The drawing under review shows one solid part. Ordinate dimensions are in mm from its lowest x, y, z. A direction names the side the tool comes from. Give positions to 0.01 mm unless a question says otherwise; leave off trailing zeros. Loops run counter-clockwise (first coordinate to the right, second up) from the corner with the lowest first, then second, coordinate; pieces in that order, holes last. Notation, with made-up numbers: (38.25, 62.25) -> (90.25, 62.25) arc R26 ccw to (90.25, 100.25) -> close; hole circle Ø6 at (-21.5, 8). An arc over 180 degrees is marked (long way). Answer in a Markdown table with one row per item. Add a question column.
(1) Consider section C-C on z = 15.75. Write out the cut boundary in (x, y), then the cut area to 4 significant figures.
(2) For the marked faces 1 and 2, list the 3-axis set-ups (+Z, -Z, +X, -X, +Y, -Y) from which the entire face can be reached by the end or side of a thin tool; tool diameter is ignored.
(3) Consider section D-D on y = 77.5. Write out the cut boundary in (x, z), then the cut area to 3 significant figures.
(4) For pin 1 (19 mm diameter, centred on x = 47, y = 59.5, fed in from +Z); pin 2 (2.5 mm diameter, centred on x = 18, z = 3.5, fed in from -Y); pin 3 (10.5 mm diameter, centred on y = 94, z = 6, fed in from +X), all flat-tipped, find the tip position at first contact; note any pin that passes through.
(5) For line 1 (X direction, y = 70.5, z = 14.5); line 2 (X direction, y = 79, z = 1.5); line 3 (Y direction, x = 19, z = 1.25), list the stretches that pass through material, from the lowest coordinate up.
(6) Draft analysis for pull direction X (two halves, no side actions). For the marked faces 3, 4 and 5, state which applies: +X half, -X half, draft (parallel to the pull), parting line (faces both ways), or undercut.
(7) Consider section B-B on y = 99. Write out the cut boundary in (x, z).
(8) Consider section A-A on z = 2. Write out the cut boundary in (x, y).
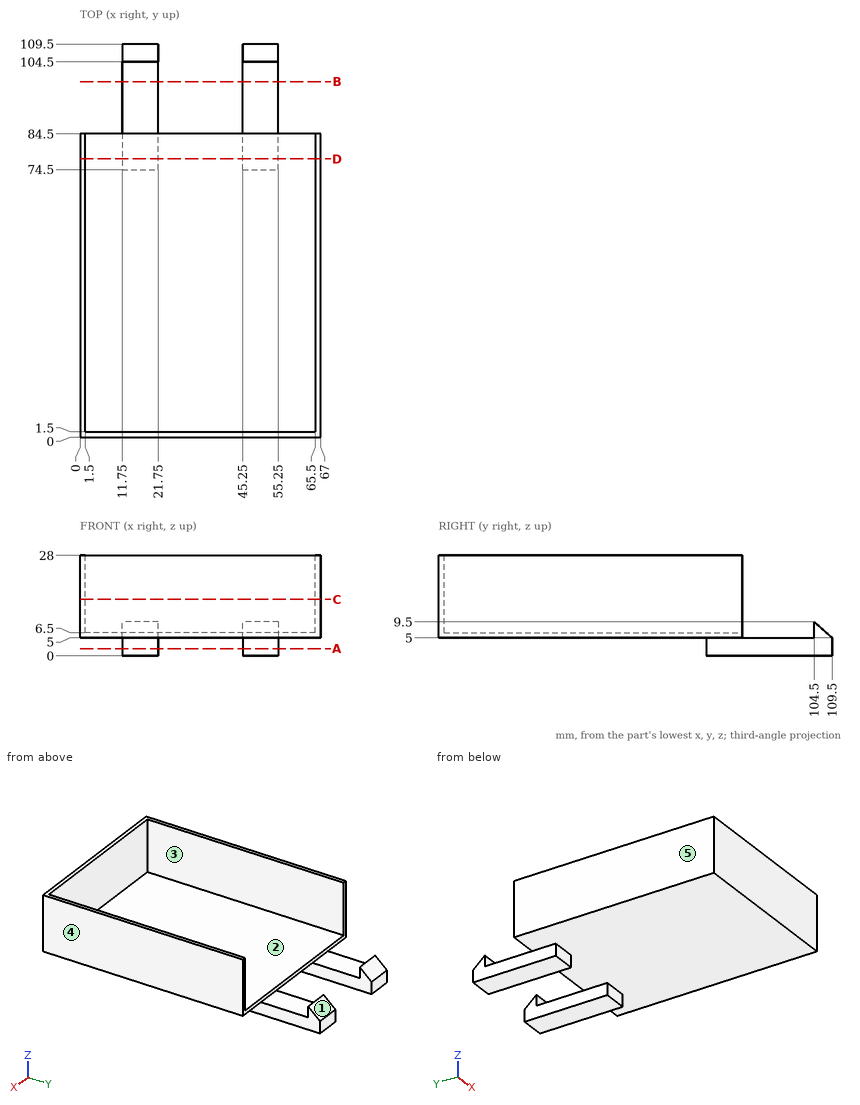
Values follow:
| question | item | result |
|---|---|---|
| 1 | outline | (0, 0) -> (67, 0) -> (67, 84.5) -> (65.5, 84.5) -> (65.5, 1.5) -> (1.5, 1.5) -> (1.5, 84.5) -> (0, 84.5) -> close |
| 1 | area | 349.5 mm2 |
| 2 | face 1 | +Z, +X, -X, +Y |
| 2 | face 2 | +Z |
| 3 | outline | (0, 5) -> (11.75, 5) -> (11.75, 0) -> (21.75, 0) -> (21.75, 5) -> (45.25, 5) -> (45.25, 0) -> (55.25, 0) -> (55.25, 5) -> (67, 5) -> (67, 28) -> (65.5, 28) -> (65.5, 6.5) -> (1.5, 6.5) -> (1.5, 28) -> (0, 28) -> close |
| 3 | area | 265 mm2 |
| 4 | pin 1 | z = 6.5 |
| 4 | pin 2 | y = 74.5 |
| 4 | pin 3 | x = 55.25 |
| 5 | line 1 | 0 to 1.5, 65.5 to 67 |
| 5 | line 2 | 11.75 to 21.75, 45.25 to 55.25 |
| 5 | line 3 | 74.5 to 109.5 |
| 6 | face 3 | undercut |
| 6 | face 4 | +X half |
| 6 | face 5 | -X half |
| 7 | outline | (11.75, 0) -> (21.75, 0) -> (21.75, 5) -> (11.75, 5) -> close; (45.25, 0) -> (55.25, 0) -> (55.25, 5) -> (45.25, 5) -> close |
| 8 | outline | (11.75, 74.5) -> (21.75, 74.5) -> (21.75, 109.5) -> (11.75, 109.5) -> close; (45.25, 74.5) -> (55.25, 74.5) -> (55.25, 109.5) -> (45.25, 109.5) -> close |
